Source: CAD feature listing. Evaluate the final solid. Frame: model axes, mm. Face numbers are marked on the shaded views. A direction names the side the tool comes from. Give positions to 0.01 mm unless a question says otherwise; leave off trailing zeros. Loops run counter-clockwise (first coordinate to the right, second up) from the corner with the lowest first, then second, coordinate; pieces in that order, holes last. Notation, with made-up numbers: (5.5, 32.25) - (32.5, 32.25) arc R9 ccw to (32.5, 48.25) - close; hole circle Ø9 at (63, 60). An arc over 180 degrees is marked (long way). Write each question's results on one line, items separated by ' | '. Start each with the question number.
(1) Contact query for flat-ended pins moving along their axis: pin 1 (3 mm diameter, centred on x = 6, z = 24, fed in from -Y); pin 2 (8 mm diameter, centred on x = 2, y = 0, fed in from +Z); pin 3 (2 mm diameter, centred on x = -1.5, z = 22.5, fed in from +Y). Output: stop coordinate, or through.
(2) Cut plane A-A on x = 0. Return the cut outline in (y, z).
(3) Pull-direction query (Y, two-part tool) for the marked faces 1, 2 and 3; classes: pulls with the +Y half, pulls with the -Y half, needs draft (parallel to the pull), parting line crosses it, or undercut.
(4) Cut plane C-C on z = 41.5. Return the cut outline in (x, y).
(5) Reachability of the marked faces 4 and 5 from +Z, -Z, +X, -X, +Y, -Y: full face, straight path, thin tool, end or side. Return the list, or none.
(6) Material intervals for line 1 along Y through (x, z) = (0, 14.5); line 2 along Y through (x, z) = (0, 26); line 3 along Y through (x, z) = (-1.75, 10), sorted ascending. Write a range as [from, to].
from build123d import *

# Parameters (mm, degrees)
F0_R        = 5
F0_R_2      = 3.5
F1_DEPTH    = 8
F2_R        = 8
F2_R_2      = 6.75
F2_R_3      = 5
F2_R_4      = 3.5
F2_R_5      = 2
F2_R_6      = 1.5
F3_DEPTH    = 1
F4_DEPTH    = 50
F5_DEPTH    = 25
F6_S5_R     = 1.5
F6_T6_DEPTH = 8
F7_R        = 2
F9_R        = 2


# Not quite as in the source:
# - a fillet or chamfer that OpenCascade refuses, or shapes differently, is made with other operations: its cross-section is extruded or revolved along the edge and cut away or added


with BuildPart() as f1:
    # F0 (on Top) → F1 (new body)
    with BuildSketch(Plane.XY):
        Circle(F0_R)
        Circle(F0_R_2, mode=Mode.SUBTRACT)
    extrude(amount=F1_DEPTH)

    # F2 (on face) → F3 (join)
    with BuildSketch(Plane.XY.offset(8)):
        Circle(F2_R)
        Circle(F2_R_2, mode=Mode.SUBTRACT)
        Circle(F2_R_2)
        Circle(F2_R_3, mode=Mode.SUBTRACT)
        Circle(F2_R_3)
        Circle(F2_R_4, mode=Mode.SUBTRACT)
        Circle(F2_R_4)
        Circle(F2_R_5, mode=Mode.SUBTRACT)
        Circle(F2_R_5)
        Circle(F2_R_6, mode=Mode.SUBTRACT)
    extrude(amount=F3_DEPTH)

    # F2 (on face) → F4 (join)
    with BuildSketch(Plane.XY.offset(8)):
        Circle(F2_R)
        Circle(F2_R_2, mode=Mode.SUBTRACT)
    extrude(amount=F4_DEPTH)

    # F2 (on face) → F5 (join)
    with BuildSketch(Plane.XY.offset(8)):
        Circle(F2_R_5)
        Circle(F2_R_6, mode=Mode.SUBTRACT)
    extrude(amount=F5_DEPTH)

    # F6: chamfer of 8 x 3 on 1 edges, made by hand


with BuildPart() as f6_tool2:
    # F6_s3 → F6_t4 (revolve)
    with BuildSketch(Plane.XZ):
        Polygon((0.5, 8), (3.5, 0), (3.5, 8), align=None)
    revolve(axis=Axis((0, 0, 8), (0, 0, 1)))

    # F6_s5 → F6_t6 (cut, symmetric)
    with BuildSketch(Plane.XY.offset(4)):
        Circle(F6_S5_R)
    extrude(amount=F6_T6_DEPTH, both=True, mode=Mode.SUBTRACT)

    split(bisect_by=Plane.XY, keep=Keep.TOP)


with BuildPart() as f1_1:
    add(f1.part)

    # F6_t1: union F6_tool2
    add(f6_tool2.part)

    # F7
    f7_edges = [f1_1.edges().sort_by_distance(p)[0] for p in [
        (-2, 0, 9),
    ]]
    fillet(f7_edges, radius=F7_R)

    # F8: chamfer of 1 x 10 on 1 edges, made by hand

    # F8_s1 → F8_t2 (revolve, cut)
    with BuildSketch(Plane.XZ):
        Polygon((2, 23), (1, 33), (2, 33), align=None)
    revolve(axis=Axis((0, 0, 33), (0, 0, 1)), mode=Mode.SUBTRACT)

    # F9
    f9_edges = [f1_1.edges().sort_by_distance(p)[0] for p in [
        (-6.75, 0, 9),
    ]]
    fillet(f9_edges, radius=F9_R)


solid = f1_1.part
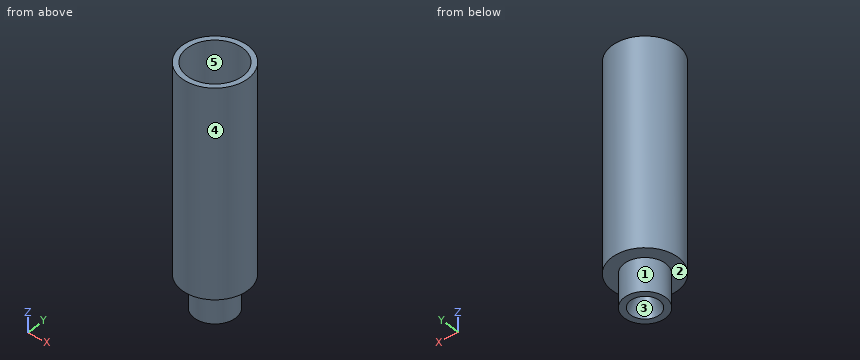
Ans:
1) pin 1: y = -6.61 | pin 2: z = 28 | pin 3: y = 7.98
2) outline: (-8, 8) - (-5, 8) - (-5, 0) - (-3.5, 0) - (-1.5, 5.33) - (-1.5, 28) - (-2, 23) - (-2, 11) arc R2 cw to (-4, 9) - (-4.75, 9) arc R2 cw to (-6.75, 11) - (-6.75, 58) - (-8, 58) - close; (1.5, 5.33) - (3.5, 0) - (5, 0) - (5, 8) - (8, 8) - (8, 58) - (6.75, 58) - (6.75, 11) arc R2 cw to (4.75, 9) - (4, 9) arc R2 cw to (2, 11) - (2, 23) - (1.5, 28) - close
3) face 1: parting line crosses it | face 2: needs draft | face 3: undercut
4) outline: circle Ø16 at (0, 0); hole circle Ø13.5 at (0, 0)
5) face 4: +Z, -Z | face 5: +Z
6) line 1: [-8, -6.75], [-2, -1.5], [1.5, 2], [6.75, 8] | line 2: [-8, -6.75], [-1.7, -1.5], [1.5, 1.7], [6.75, 8] | line 3: [-7.81, -6.24], [-1.44, 1.44], [6.24, 7.81]
